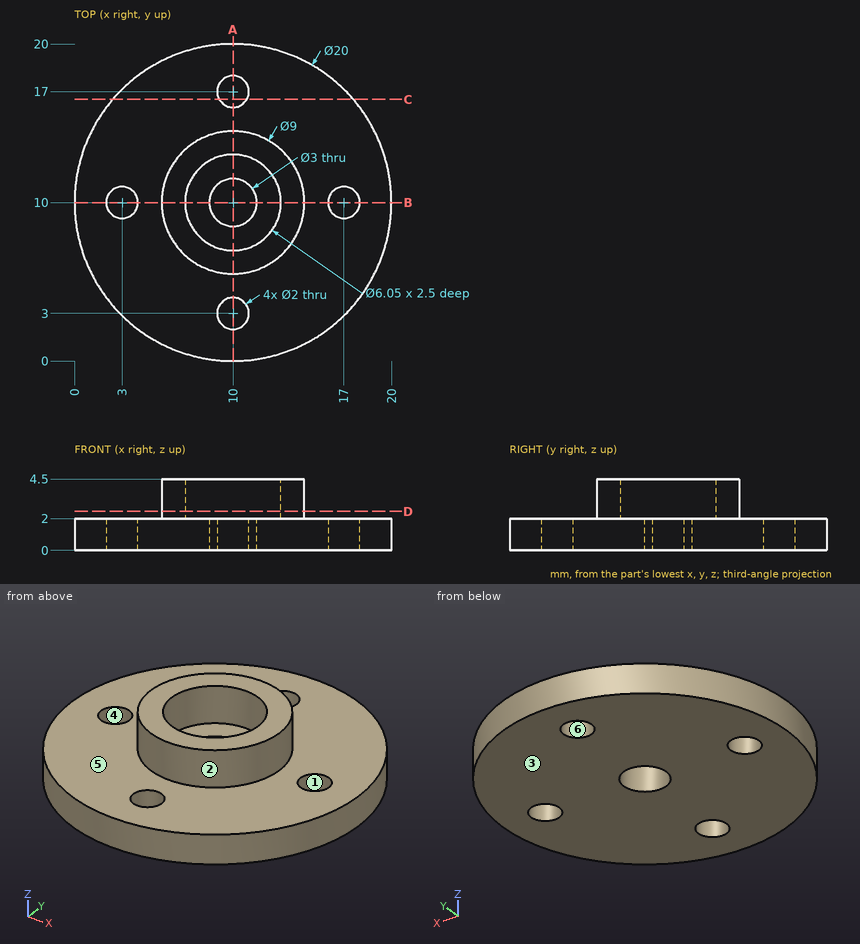
Can you work these out from the drawing? Everything is in mm from the part's minimum corner. A direction names the side the tool comes from. Round coordinates to 2 decimals unless told otherwise and drop trailing zeros. Write each loop counter-clockwise with the first axis right and the second up, starting at its lowest first coordinate (ties: lowest second). Pieces come first, ordered by that corner, then holes. Notation, with made-up numbers: (36.25, -34.75) - (84.25, -34.75) arc R10 cw to (84.25, -23.75) - close; hole circle Ø4 at (62.5, 81). An arc over 180 degrees is marked (long way). Put each result on its own line as item: value. Start each with the question number.
(1) I want a section at D-D, the plane z = 2.45. Please give me the cut outline in (x, y) (3 decimals), plus the area to 3 significant figures.
(2) I want a section at C-C, the plane y = 16.5. Please give me the cut outline in (x, z), plus the area to 3 significant figures.
(3) For the marked faces 5 and 6, which set-ups out of +Z, -Z, +X, -X, +Y, -Y let a thin tool reach every point of the face, with its end or its side?
(4) I need wall thicknesses on probe 1 along Y at (x, z) = (10, 1.1); probe 2 along Z at (x, y) = (5, 9.5); probe 3 along X at (y, z) = (11.25, 0.55). Which ranges of each line are inside material? Lowest first, please.
(5) I want a section at A-A, the plane x = 10. Please give me the cut outline in (y, z) (3 decimals), plus the area to 3 significant figures.
(6) Thinking about a two-plate mould opening in X: for the marked faces 1, 2, 3 and 4, which applies, released by +X, released by -X, zero draft, split by the parting line, or undercut?
(7) Will this pin go through, and if not, where does the flat tip stop? pin 1 (5 mm diameter, centred on x = 10.5, y = 17.5, fed in from +Z).
Here are the results:
1. outline: circle Ø9 at (10, 10); hole circle Ø6.05 at (10, 10)
1. area: 34.9 mm^2
2. outline: (2.4, 0) - (9.13, 0) - (9.13, 2) - (2.4, 2) - close; (10.87, 0) - (17.6, 0) - (17.6, 2) - (10.87, 2) - close
2. area: 26.9 mm^2
3. face 5: +Z
3. face 6: +Z, -Z
4. probe 1: y = 0 to 2, 4 to 8.5, 11.5 to 16, 18 to 20
4. probe 2: z = 0 to 2
4. probe 3: x = 0.08 to 9.17, 10.83 to 19.92
5. outline: (0, 0) - (2, 0) - (2, 2) - (0, 2) - close; (4, 0) - (8.5, 0) - (8.5, 2) - (6.975, 2) - (6.975, 4.5) - (5.5, 4.5) - (5.5, 2) - (4, 2) - close; (11.5, 0) - (16, 0) - (16, 2) - (14.5, 2) - (14.5, 4.5) - (13.025, 4.5) - (13.025, 2) - (11.5, 2) - close; (18, 0) - (20, 0) - (20, 2) - (18, 2) - close
5. area: 33.4 mm^2
6. face 1: undercut
6. face 2: split by the parting line
6. face 3: zero draft
6. face 4: undercut
7. pin 1: stops at z = 2
